Verification items for this drawing (mm, ordinates from the low corner). A direction names the side the tool comes from. Give positions to 0.01 mm unless a question says otherwise; leave off trailing zeros. Write each loop counter-clockwise with the first axis right and the second up, starting at its lowest first coordinate (ties: lowest second). Pieces come first, ordered by that corner, then holes. Notation, with made-up numbers: (19.5, -22) -> (74.5, -22) arc R29 cw to (74.5, -1) -> close; hole circle Ø4 at (-6.5, 57). An arc over 180 degrees is marked (long way). One line per item, written item: value.
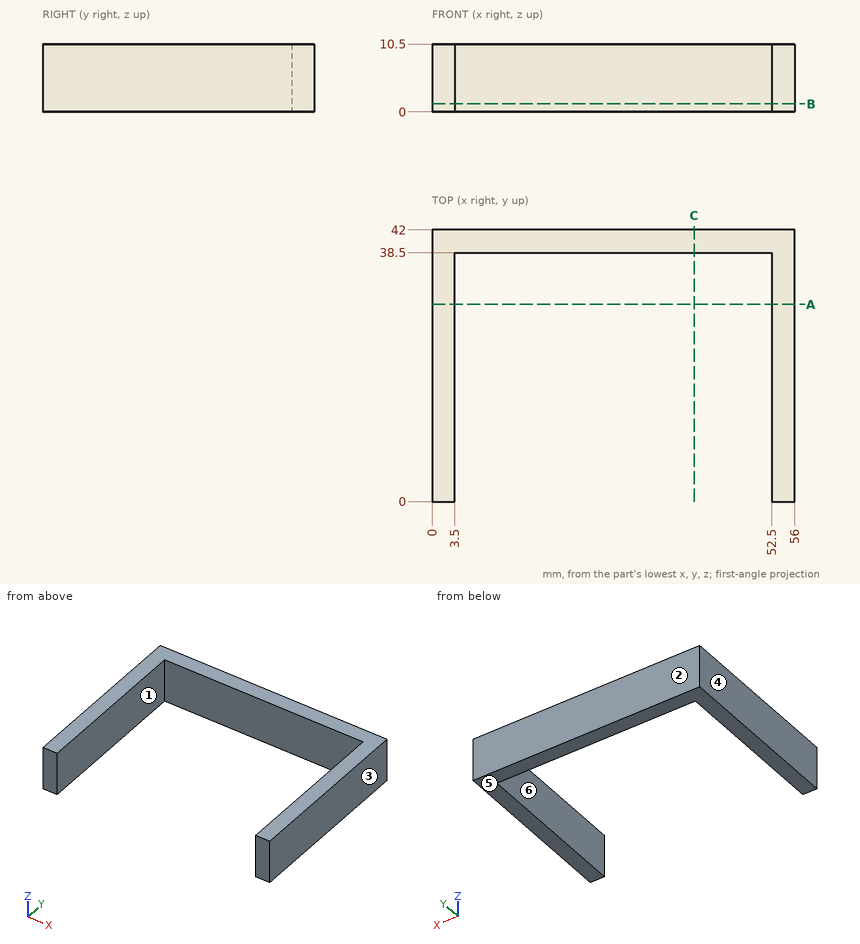
1) Sectioned sample at C-C on x = 40.5. Record the cut outline in (y, z), plus the area to 4 significant figures.
Verdict:
outline: (38.5, 0) -> (42, 0) -> (42, 10.5) -> (38.5, 10.5) -> close
area: 36.75 mm^2
2) Tool access check on the marked faces 5 and 6. Record the directions out of +Z, -Z, +X, -X, +Y, -Y that give a thin tool (end or side, any length) a straight path to the whole face; none if there is none.
Verdict:
face 5: -Z, +X, -X, +Y, -Y
face 6: +Z, -Z, -Y
3) Depth check by flat-ended pin: pin 1 Ø1 at (y, z) = (22.5, 2.5) entering from -X; pin 2 Ø1.5 at (x, z) = (22.5, 2.5) entering from -Y. Enter the tip coordinate at first touch or a pass-through.
Verdict:
pin 1: x = 0
pin 2: y = 38.5
4) Sectioned sample at B-B on z = 1.25. Record the cut outline in (x, y), plus the area to 4 significant figures.
Verdict:
outline: (0, 0) -> (3.5, 0) -> (3.5, 38.5) -> (52.5, 38.5) -> (52.5, 0) -> (56, 0) -> (56, 42) -> (0, 42) -> close
area: 465.5 mm^2
5) Scan lines: probe 1 along X at (y, z) = (17.5, 4.75); probe 2 along Y at (x, z) = (32, 5.25). Record each from-to range of solid material in increasing order.
Verdict:
probe 1: 0 to 3.5, 52.5 to 56
probe 2: 38.5 to 42
6) Mould release check, pull along X, two halves, no side actions. Record for the marked faces 1, 2, 3 and 4: released by +X, released by -X, zero draft, split by the parting line, or undercut.
Verdict:
face 1: undercut
face 2: zero draft
face 3: released by +X
face 4: released by -X
7) Sectioned sample at A-A on y = 30.5. Record the cut outline in (x, z), plus the area to 3 significant figures.
Verdict:
outline: (0, 0) -> (3.5, 0) -> (3.5, 10.5) -> (0, 10.5) -> close; (52.5, 0) -> (56, 0) -> (56, 10.5) -> (52.5, 10.5) -> close
area: 73.5 mm^2
